```python
from build123d import *

# Parameters (mm, degrees)
F1_DEPTH = 2


with BuildPart() as f1:
    # F0 (on Top) → F1 (new body)
    with BuildSketch(Plane.XY):
        Polygon((-15.224708, -0.007928), (-7.605488, -13.188947), (7.61922, -13.18102), (15.224708, 0.007928), (7.605488, 13.188947), (-7.61922, 13.18102), align=None)
        Polygon((4.384312, -11.191897), (-6.725698, -11.222334), (-13.29542, 0.143087), (-6.687111, 11.60279), (4.683197, 11.608711), (11.105834, 0), align=None, mode=Mode.SUBTRACT)
    extrude(amount=F1_DEPTH)


solid = f1.part
```
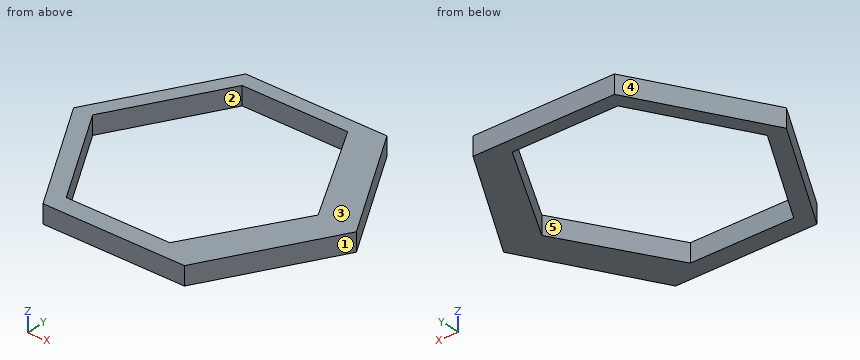
Verification items for the finished model (mm, model axes). Face numbers are marked on the shaded views. A direction names the side the tool comes from. Give positions to 0.01 mm unless a question says otherwise; leave off trailing zeros. Order: outer loops, then holes, each group sorted by start corner. A loop starts at its lowest first (then second) coordinate and runs counter-clockwise, first axis right, second up. Notation, with made-up numbers: M 60.5,44.5 L 113.5,44.5 A28 cw 113.5,80.5 Z; hole C 13.5,40.25 d3. An arc over 180 degrees is marked long. Answer in a Markdown table with one row per item. Add a question column.
Item 1: Section check D-D, the plane x = 12. Enter the section's corners in (y, z).
Item 2: Section check C-C, the plane x = -8.5. Enter the section's corners in (y, z).
Item 3: Tool access check on the marked faces 4 and 5. Record the directions out of +Z, -Z, +X, -X, +Y, -Y that give a thin tool (end or side, any length) a straight path to the whole face; none if there is none.
Item 4: Mould release check, pull along Y, two halves, no side actions. Record for the marked faces 1, 2 and 3: released by +Y, released by -Y, zero draft, split by the parting line, or undercut.
Item 5: Section check A-A, the plane z = 1.3. Enter the section's corners in (x, y).
Item 6: Scan lines: probe 1 along Y at (x, z) = (-4.5, 1.8); probe 2 along X at (y, z) = (3.5, 0.45); probe 3 along X at (y, z) = (5, 0.95). Record each from-to range of solid material in increasing order. Write a range as from..to.
Item 7: Section check B-B, the plane y = -7.25. Enter the section's corners in (x, z), and give its area (3 significant figures).
Item 8: Gauge pin test, flat ends, axial feed: pin 1 (8 mm diameter, centred on x = -10.5, y = -9, fed in from +Z); pin 2 (1 mm diameter, centred on x = -2.5, z = 0.5, fed in from +Y). Record the tip position at first contact, or that the pin passes through.
Filled sheet:
| question | item | result |
|---|---|---|
| 1 | outline | M -5.58,0 L 5.59,0 L 5.59,2 L -5.58,2 Z |
| 2 | outline | M -11.64,0 L -8.15,0 L -8.15,2 L -11.64,2 Z; M 8.46,0 L 11.65,0 L 11.65,2 L 8.46,2 Z |
| 3 | face 4 | +Z, -Z, -X, +Y |
| 3 | face 5 | +Z, -Z |
| 4 | face 1 | released by -Y |
| 4 | face 2 | undercut |
| 4 | face 3 | zero draft |
| 5 | outline | M -15.22,-0.01 L -7.61,-13.19 L 7.62,-13.18 L 15.22,0.01 L 7.61,13.19 L -7.62,13.18 Z; hole M -13.3,0.14 L -6.73,-11.22 L 4.38,-11.19 L 11.11,0 L 4.68,11.61 L -6.69,11.6 Z |
| 6 | probe 1 | y = -13.19..-11.22, 11.6..13.18 |
| 6 | probe 2 | x = -13.2..-11.36, 9.17..13.21 |
| 6 | probe 3 | x = -12.34..-10.49, 8.34..12.34 |
| 7 | outline | M -11.04,0 L -9.02,0 L -9.02,2 L -11.04,2 Z; M 6.75,0 L 11.04,0 L 11.04,2 L 6.75,2 Z |
| 7 | area | 12.6 mm^2 |
| 8 | pin 1 | stops at z = 2 |
| 8 | pin 2 | stops at y = 13.18 |
